```python
from build123d import *

# Parameters (mm, degrees)
BOSS_EXTRUDE1_DEPTH = 6.35
SKETCH2_W           = 2.54
SKETCH2_H           = 2.54
BOSS_EXTRUDE2_DEPTH = 2.54
BOSS_EXTRUDE3_DEPTH = 7.62


with BuildPart() as part:
    # Sketch1 → Boss-Extrude1 (new body)
    with BuildSketch(Plane.XY):
        Polygon((6.35, -3.429), (-6.35, -3.429), (-6.35, 3.429), (-2.54, 3.429), (-2.54, -2.159), (2.54, -2.159), (2.54, 3.429), (6.35, 3.429), align=None)
    extrude(amount=BOSS_EXTRUDE1_DEPTH)

    # Sketch2 → Boss-Extrude2 (add)
    with BuildSketch(Plane.XZ.offset(3.429)):
        with Locations((0, 3.175)):
            Rectangle(SKETCH2_W, SKETCH2_H)
    extrude(amount=BOSS_EXTRUDE2_DEPTH)

    # Sketch3 → Boss-Extrude3 (add)
    with BuildSketch(Plane.XZ.offset(3.429)):
        with BuildLine():
            Line((-4.711095298, 1.905), (-4.711095298, 4.445))
            ThreePointArc((-4.711095298, 4.445), (-3.441095298, 5.715), (-2.171095298, 4.445))
            Line((-2.171095298, 4.445), (-2.171095298, 1.905))
            ThreePointArc((-2.171095298, 1.905), (-3.441095298, 0.635), (-4.711095298, 1.905))
        make_face()
        with BuildLine():
            Line((4.711095298, 1.905), (4.711095298, 4.445))
            ThreePointArc((4.711095298, 4.445), (3.441095298, 5.715), (2.171095298, 4.445))
            Line((2.171095298, 4.445), (2.171095298, 1.905))
            ThreePointArc((2.171095298, 1.905), (3.441095298, 0.635), (4.711095298, 1.905))
        make_face()
    extrude(amount=BOSS_EXTRUDE3_DEPTH)


solid = part.part
```
For this review, take the finished solid that the model builds, in its own axes (mm). A direction names the side the tool comes from. Coordinates: 2 decimals unless noted, no trailing zeros. Loops run counter-clockwise (first coordinate to the right, second up) from the corner with the lowest first, then second, coordinate; pieces in that order, holes last.
1. Insertion check: P1, Ø2, axis at y = -7, z = 3.5, coming from the -X side; P2, Ø0.8, axis at y = -5, z = 3, coming from the +X side; P3, Ø0.8, axis at x = 0, z = 2.5, coming from the -Y side. Each pin has a flat end and moves straight along its axis. Give the tip position at first contact, or say it passes through.
2. Add section C-C, the plane x = 0.5. Give the boundary of the cut face in (y, z) (3 decimals), then the cut area to 3 significant figures.
3. Add section D-D, the plane y = -7.5. Give the boundary of the cut face in (x, z) (3 decimals).
4. For line 1 (X direction, y = -5.25, z = 2.25); line 2 (X direction, y = 2.25, z = 4); line 3 (X direction, y = -7.75, z = 4.5), list the stretches that pass through material, from the lowest coordinate up.
5. For faces 1 (the flat face through (0, -2.159, 3)), 2 (the cylindrical face through (3.469, -7.186, 5.715)), 3 (the cylindrical face through (3.413, -7.186, 0.635)), 4 (the flat face through (4.711, -7, 3)), 5 (the flat face through (-4.711, -7, 3)), list the 3-axis set-ups (+Z, -Z, +X, -X, +Y, -Y) from which the entire face can be reached by the end or side of a thin tool; tool diameter is ignored.
6. Mouldability with a two-part tool opening along X and no side actions: class faces 6 (the flat face through (-3, -11.049, 3)), 7 (the flat face through (6.35, 0, 3)), 8 (the flat face through (1.27, -5, 3)) as +X half, -X half, draft (parallel to the pull), parting line (faces both ways), or undercut.
7. Add section A-A, the plane y = 0.75. Give the boundary of the cut face in (x, z).
8. Add section B-B, the plane z = 4. Give the boundary of the cut face in (x, y).
Result:
1. P1: stops at x = -4.71
1. P2: stops at x = 4.71
1. P3: stops at y = -5.97
2. outline: (-5.969, 1.905) - (-3.429, 1.905) - (-3.429, 0) - (-2.159, 0) - (-2.159, 6.35) - (-3.429, 6.35) - (-3.429, 4.445) - (-5.969, 4.445) - close
2. area: 14.5 mm2
3. outline: (-4.711, 1.905) arc R1.27 ccw to (-2.171, 1.905) - (-2.171, 4.445) arc R1.27 ccw to (-4.711, 4.445) - close; (2.171, 1.905) arc R1.27 ccw to (4.711, 1.905) - (4.711, 4.445) arc R1.27 ccw to (2.171, 4.445) - close
4. line 1: x = -4.71 to -2.17, -1.27 to 1.27, 2.17 to 4.71
4. line 2: x = -6.35 to -2.54, 2.54 to 6.35
4. line 3: x = -4.71 to -2.17, 2.17 to 4.71
5. face 1: +Z, -Z, +Y
5. face 2: +Z, -Y
5. face 3: -Z, -Y
5. face 4: +Z, -Z, +X, -Y
5. face 5: +Z, -Z, -X, -Y
6. face 6: draft
6. face 7: +X half
6. face 8: undercut
7. outline: (-6.35, 0) - (-2.54, 0) - (-2.54, 6.35) - (-6.35, 6.35) - close; (2.54, 0) - (6.35, 0) - (6.35, 6.35) - (2.54, 6.35) - close
8. outline: (-6.35, -3.43) - (-4.71, -3.43) - (-4.71, -11.05) - (-2.17, -11.05) - (-2.17, -3.43) - (-1.27, -3.43) - (-1.27, -5.97) - (1.27, -5.97) - (1.27, -3.43) - (2.17, -3.43) - (2.17, -11.05) - (4.71, -11.05) - (4.71, -3.43) - (6.35, -3.43) - (6.35, 3.43) - (2.54, 3.43) - (2.54, -2.16) - (-2.54, -2.16) - (-2.54, 3.43) - (-6.35, 3.43) - close
